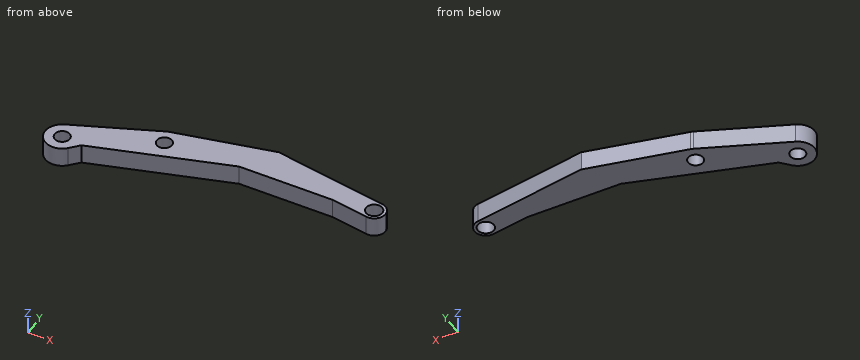
```python
from build123d import *

# Parameters (mm, degrees)
F0_R     = 1
F0_R_2   = 1.075
F1_DEPTH = 2.6


with BuildPart() as f1:
    # F0 (on Top) → F1 (new body)
    with BuildSketch(Plane.XY):
        with BuildLine():
            ThreePointArc((-4.746486, 4.808329), (-5.079824, 1.124576), (-1.822392, 2.876799))
            ThreePointArc((-1.822392, 2.876799), (-2.614969, 4.520158), (-4.394433, 4.923045))
            ThreePointArc((-4.394433, 4.923045), (-4.572993, 4.873462), (-4.746486, 4.808329))
        make_face()
        with Locations((-3.922381, 2.876799)):
            Circle(F0_R, mode=Mode.SUBTRACT)
        with BuildLine():
            ThreePointArc((-4.394433, 4.923045), (-2.614969, 4.520158), (-1.822392, 2.876799))
            ThreePointArc((-1.822392, 2.876799), (-5.079824, 1.124576), (-4.746486, 4.808329))
            Line((-4.746486, 4.808329), (-15.782993, 0.099507))
            ThreePointArc((-15.782993, 0.099507), (-13.659897, -0.09261), (-12.65002, -1.97))
            ThreePointArc((-12.65002, -1.97), (-12.802118, -2.78321), (-13.237851, -3.486475))
            Line((-13.237851, -3.486475), (-12.155538, -2.30018))
            Line((-12.155538, -2.30018), (5.849769, 3.333367))
            Line((5.849769, 3.333367), (18.365619, 3.333367))
            Line((18.365619, 3.333367), (23.356251, 2.544399))
            ThreePointArc((23.356251, 2.544399), (22.108876, 4.260224), (23.824702, 5.507599))
            Line((23.824702, 5.507599), (8.583845, 7.917022))
            Line((8.583845, 7.917022), (-4.394433, 4.923045))
        make_face()
        with BuildLine():
            ThreePointArc((-12.65002, -1.97), (-13.659897, -0.09261), (-15.782993, 0.099507))
            ThreePointArc((-15.782993, 0.099507), (-16.73485, -3.272267), (-13.237851, -3.486475))
            ThreePointArc((-13.237851, -3.486475), (-12.802118, -2.78321), (-12.65002, -1.97))
        make_face()
        with Locations((-14.90002, -1.97)):
            Circle(F0_R, mode=Mode.SUBTRACT)
        with BuildLine():
            ThreePointArc((25.090476, 4.025999), (24.730945, 5.000335), (23.824702, 5.507599))
            ThreePointArc((23.824702, 5.507599), (22.108876, 4.260224), (23.356251, 2.544399))
            ThreePointArc((23.356251, 2.544399), (24.564812, 2.88553), (25.090476, 4.025999))
        make_face()
        with Locations((23.590476, 4.025999)):
            Circle(F0_R_2, mode=Mode.SUBTRACT)
    extrude(amount=F1_DEPTH)


solid = f1.part
```
The listing builds one solid part. Answer for the finished solid, in the listing's coordinates (mm). Coordinates: 2 decimals unless noted, no trailing zeros. Loops run counter-clockwise (first coordinate to the right, second up) from the corner with the lowest first, then second, coordinate; pieces in that order, holes last. Notation, with made-up numbers: (50.5, 63) -> (63.5, 63) arc R25 cw to (63.5, 83) -> close; hole circle Ø9 at (-21.75, 85). An arc over 180 degrees is marked (long way). Return JSON: item names as keys, results as strings. Group by question number.
(1) Given pin 1 Ø1 at (x, z) = (7.5, 1.5) entering from +Y; pin 2 Ø1.3 at (x, z) = (13, 1.5) entering from -Y, each flat-ended and moving along its own axis, determine where each tip first touches the part or whether it passes through.
(2) A cutting plane is placed at B-B on x = 20. Write down the section's boundary in (y, z).
(3) A cutting plane is placed at A-A on z = 0.7. Count the separate pieces of the cut face and the enclosed holes in it, and give its area (3 significant figures).
(4) Find the intervals of material crossed by probe 1 along X at (y, z) = (3.5, 1.8); probe 2 along X at (y, z) = (4.75, 1.4); probe 3 along Y at (x, z) = (-8, 0.85), in increasing order. Write a range as from..to.
The answers:
{
 "1": {"pin 1": "stops at y = 7.78", "pin 2": "stops at y = 3.33"},
 "2": {"outline": "(3.07, 0) -> (6.11, 0) -> (6.11, 2.6) -> (3.07, 2.6) -> close"},
 "3": {"separate pieces": "1", "enclosed holes": "3", "area": "158 mm^2"},
 "4": {"probe 1": "x = -7.81..-4.7, -3.14..22.65, 24.53..25", "probe 2": "x = -4.88..22.8, 24.39..24.9", "probe 3": "y = -1..3.42"}
}
